Source: CAD feature listing. Evaluate the final solid. Frame: model axes, mm. A direction names the side the tool comes from. Give positions to 0.01 mm unless a question says otherwise; leave off trailing zeros. Order: outer loops, then holes, each group sorted by start corner. A loop starts at its lowest first (then second) coordinate and runs counter-clockwise, first axis right, second up.
Autodesk Inventor part; units mm, degrees
ref_plane "YZ Plane" through (0, 0, 0) normal (1, 0, 0) x (0, 1, 0)
ref_plane "XZ Plane" through (0, 0, 0) normal (0, 1, 0) x (-1, 0, 0)
ref_plane "XY Plane" through (0, 0, 0) normal (0, 0, 1) x (1, 0, 0)
sketch "Sketch1" plane through (0, 0, 0) normal (0, 0, 1) x (1, 0, 0)
  line L0 (0, 0) -> (25.4, 0)
  line L1 (25.4, 0) -> (25.4, 25.4)
  line L2 (25.4, 25.4) -> (0, 25.4)
  line L3 (0, 25.4) -> (0, 0)
  line L4 (3.175, 22.225) -> (22.225, 22.225)
  line L5 (22.225, 22.225) -> (22.225, 3.175)
  line L6 (22.225, 3.175) -> (3.175, 3.175)
  line L7 (3.175, 3.175) -> (3.175, 22.225)
  dimension "d0" = 25.4
  dimension "d1" = 25.4
  dimension "d2" = 3.175
extrude "Extrusion1" add sketch "Sketch1" against normal blind 355.6
sketch "Sketch2" plane through (0, 0, 0) normal (-1, 0, 0) x (0, 0, 1)
  line L0 (-355.6, 25.4) -> (-355.6, 0)
  line L1 (0, 25.4) -> (0, 0)
  point P0 (-266.7, 12.7)
  point P1 (-241.3, 12.7)
  point P2 (-215.9, 12.7)
  point P3 (-12.7, 12.7)
  point P4 (-38.1, 12.7)
  point P5 (-63.5, 12.7)
  dimension "d5" = 88.9
  dimension "d6" = 25.4
  dimension "d7" = 25.4
  dimension "d8" = 25.4
  dimension "d9" = 25.4
  dimension "d10" = 12.7
hole "Hole1" at (0, 12.7, -266.7) at (0, 12.7, -241.3) at (0, 12.7, -215.9) at (0, 12.7, -12.7) at (0, 12.7, -38.1) at (0, 12.7, -63.5) direction (1, 0, 0) diameter 6.35 depth 25.4 tip angle 118
sketch "Sketch3" plane through (0, 25.4, 0) normal (0, 1, 0) x (1, 0, 0)
  line L0 (25.4, 355.6) -> (0, 355.6)
  point P0 (12.7, 342.9)
  point P1 (12.7, 317.5)
  point P2 (12.7, 292.1)
  dimension "d18" = 25.4
  dimension "d19" = 25.4
  dimension "d20" = 12.7
hole "Hole2" at (12.7, 25.4, -342.9) at (12.7, 25.4, -317.5) at (12.7, 25.4, -292.1) direction (0, -1, 0) diameter 6.35 depth 25.4 tip angle 118
properties part number "10 inch side piece"
1) Reachability of faces 5 (the face through (13, 22.225, -175)), 6 (the face through (1.6, 15.5, -11.2)) from +Z, -Z, +X, -X, +Y, -Y: full face, straight path, thin tool, end or side. Return the list, or none.
Checks:
face 5: +Z, -Z
face 6: +X, -X
2) Section query A-A on x = 12.7. State how many separate pieces and enclosed holes the cut face has, and give its area (3 significant figures).
Checks:
separate pieces: 8
enclosed holes: 0
area: 2,140 mm2
3) Pull-direction query (X, two-part tool) for faces 1 (the face through (12.56, 1.57, -295.27)), 2 (the face through (0, 13, -175)), 3 (the face through (13, 3.175, -175)), 4 (the face through (13, 25.4, -175)); classes: +X half, -X half, draft (parallel to the pull), parting line (faces both ways), or undercut.
Checks:
face 1: undercut
face 2: -X half
face 3: undercut
face 4: draft
4) Section query C-C on z = -124.5. Output: boundary loops of the cut face in (x, y) (3 decimals).
Checks:
outline: (0, 0) - (25.4, 0) - (25.4, 25.4) - (0, 25.4) - close; hole (3.175, 3.175) - (22.225, 3.175) - (22.225, 22.225) - (3.175, 22.225) - close
5) First-contact query: pin 1 Ø5.5 at (x, z) = (12.7, -292.1) entering from -Y. Flat tip, straight axial feed; report the tip coordinate or a pass-through.
Checks:
pin 1: passes through
6) Section query B-B on z = -292.1. Output: boundary loops of the cut face in (x, y) (3 decimals).
Checks:
outline: (0, 0) - (9.525, 0) - (9.525, 3.175) - (3.175, 3.175) - (3.175, 22.225) - (9.525, 22.225) - (9.525, 25.4) - (0, 25.4) - close; (15.875, 0) - (25.4, 0) - (25.4, 25.4) - (15.875, 25.4) - (15.875, 22.225) - (22.225, 22.225) - (22.225, 3.175) - (15.875, 3.175) - close
7) Ray query, L1, parallel to Z at x = 12.7, y = 1.8 (3 decimals); L2, parallel to X at y = 24.75, z = -292.1 (3 decimals); L3, parallel to Y at x = 21, z = -240.5 (3 decimals). Return the intervals inside material, ascending.
Checks:
L1: z = -355.6 to -346.075, -339.725 to -320.675, -314.325 to -295.275, -288.925 to 0
L2: x = 0 to 9.525, 15.875 to 25.4
L3: y = 0 to 3.175, 22.225 to 25.4
